Could you check a few things on this model? Use its own coordinates, in mm. A direction names the side the tool comes from. Coordinates: 2 decimals unless noted, no trailing zeros. Order: outer loops, then holes, each group sorted by start corner. A loop starts at its lowest first (then second) coordinate and runs counter-clockwise, first axis right, second up. Notation, with made-up numbers: (79.5, 59.5) -> (127.5, 59.5) arc R9 ccw to (127.5, 76.5) -> close; hole circle Ø10 at (-5.75, -37.5). An arc over 180 degrees is marked (long way). Use a Markdown table: item, result. Add a question column.
1) Which directions (+Z, -Z, +X, -X, +Y, -Y) give clear straight access to the entire face, cutting with the end or side of a thin tool? Please do faces 1 (the flat face through (9.657, 24, 3)), 2 (the flat face through (-7, 16, 6)).
2) If we section it at C-C (x = -2): Write out the boundary of the cut face in (y, z), plus the area to 3 significant figures.
3) If I drill on L1, parallel to X at y = 30.5, z = 5.15; L2, parallel to Y at x = -14.5, z = 5.35; L3, parallel to X at y = 3, z = 2.8, over which ranges is the centre line in solid material (lowest first)? Write a range as [from, to].
4) If we section it at A-A (y = 15): Write out the boundary of the cut face in (x, z), plus the area to 3 significant figures.
5) If we section it at B-B (z = 3.55): Write out the boundary of the cut face in (x, y), plus the area to 3 significant figures.
6) Will this pin go through, and if not, where does the flat tip stop? pin 1 Ø6 at (x, y) = (16, 24.5) entering from -Z.
7) Thinking about a two-plate mould opening in X: for faces 3 (the cylindrical face through (10.56, 44.37, 2.96)), 4 (the flat face through (-11, 45.227, 3)), 5 (the flat face through (-17.343, 14, 3)), which applies, +X half, -X half, draft (parallel to the pull), parting line (faces both ways), or undercut?
```python
from build123d import *

# Parameters (mm, degrees)
F1_DEPTH = 6


with BuildPart() as f1:
    # F0 (on Top) → F1 (new body)
    with BuildSketch(Plane.XY):
        with BuildLine():
            Line((-17.343273, -14.773325), (22.656727, -14.773325))
            Line((22.656727, -14.773325), (22.656727, 42.226675))
            ThreePointArc((22.656727, 42.226675), (21.778048, 44.347996), (19.656727, 45.226675))
            Line((19.656727, 45.226675), (12.656727, 45.226675))
            ThreePointArc((12.656727, 45.226675), (10.535407, 44.347996), (9.656727, 42.226675))
            Line((9.656727, 42.226675), (9.656727, 5.226675))
            ThreePointArc((9.656727, 5.226675), (2.656727, -1.773325), (-4.343273, 5.226675))
            Line((-4.343273, 5.226675), (-4.343273, 42.226675))
            ThreePointArc((-4.343273, 42.226675), (-5.221952, 44.347996), (-7.343273, 45.226675))
            Line((-7.343273, 45.226675), (-14.343273, 45.226675))
            ThreePointArc((-14.343273, 45.226675), (-16.464593, 44.347996), (-17.343273, 42.226675))
            Line((-17.343273, 42.226675), (-17.343273, -14.773325))
        make_face()
    extrude(amount=F1_DEPTH)


solid = f1.part
```
Answer sheet:
| question | item | result |
|---|---|---|
| 1 | face 1 | +Z, -Z, +Y |
| 1 | face 2 | +Z, +X, -X, +Y, -Y |
| 2 | outline | (-14.77, 0) -> (0, 0) -> (0, 6) -> (-14.77, 6) -> close |
| 2 | area | 88.6 mm2 |
| 3 | L1 | [-17.34, -4.34], [9.66, 22.66] |
| 3 | L2 | [-14.77, 45.22] |
| 3 | L3 | [-17.34, -3.98], [9.29, 22.66] |
| 4 | outline | (-17.34, 0) -> (-4.34, 0) -> (-4.34, 6) -> (-17.34, 6) -> close; (9.66, 0) -> (22.66, 0) -> (22.66, 6) -> (9.66, 6) -> close |
| 4 | area | 156 mm2 |
| 5 | outline | (-17.34, -14.77) -> (22.66, -14.77) -> (22.66, 42.23) arc R3 ccw to (19.66, 45.23) -> (12.66, 45.23) arc R3 ccw to (9.66, 42.23) -> (9.66, 5.23) arc R7 cw to (-4.34, 5.23) -> (-4.34, 42.23) arc R3 ccw to (-7.34, 45.23) -> (-14.34, 45.23) arc R3 ccw to (-17.34, 42.23) -> close |
| 5 | area | 1,760 mm2 |
| 6 | pin 1 | z = 0 |
| 7 | face 3 | undercut |
| 7 | face 4 | draft |
| 7 | face 5 | -X half |
